```python
from build123d import *

# Parameters (mm, degrees)
F0_W     = 279.4
F0_H     = 330.2
F1_DEPTH = 5.842
F2_W     = 25.4
F2_H     = 5.842
F2_W_2   = 5.842
F2_H_2   = 25.4
F2_H_3   = 38.1
F3_DEPTH = 5.842
F5_DEPTH = 5.842
F6_W     = 5.842
F6_H     = 12.7
F7_DEPTH = 5.842
F8_R     = 3.175
F9_DEPTH = 5.842


with BuildPart() as f1:
    # F0 (on Front) → F1 (new body)
    with BuildSketch(Plane.XZ):
        with Locations((25.751306051, 40.8756073241)):
            Rectangle(F0_W, F0_H)
    extrude(amount=F1_DEPTH)

    # F2 (on face) → F3 (cut, through all)
    with BuildSketch(Plane.XZ.offset(5.842)):
        with Locations((152.751306051, -121.3033926759)):
            Rectangle(F2_W, F2_H)
        with Locations((101.951306051, -121.3033926759)):
            Rectangle(F2_W, F2_H)
        with Locations((51.151306051, -121.3033926759)):
            Rectangle(F2_W, F2_H)
        with Locations((0.351306051, -121.3033926759)):
            Rectangle(F2_W, F2_H)
        with Locations((-50.448693949, -121.3033926759)):
            Rectangle(F2_W, F2_H)
        with Locations((162.530306051, -86.1243926759)):
            Rectangle(F2_W_2, F2_H_2)
        with Locations((162.530306051, -28.9743926759)):
            Rectangle(F2_W_2, F2_H_3)
        with Locations((-111.027693949, -86.1243926759)):
            Rectangle(F2_W_2, F2_H_2)
        with Locations((-111.027693949, -35.3243926759)):
            Rectangle(F2_W_2, F2_H_2)
        with Locations((-111.027693949, 15.4756073241)):
            Rectangle(F2_W_2, F2_H_2)
        with Locations((-111.027693949, 66.2756073241)):
            Rectangle(F2_W_2, F2_H_2)
        with Locations((-111.027693949, 167.8756073241)):
            Rectangle(F2_W_2, F2_H_2)
        with Locations((-111.027693949, 117.0756073241)):
            Rectangle(F2_W_2, F2_H_2)
        with Locations((-101.248693949, -121.3033926759)):
            Rectangle(F2_W, F2_H)
    extrude(amount=-F3_DEPTH, mode=Mode.SUBTRACT)

    # F4 (on face) → F5 (cut, through all)
    with BuildSketch(Plane.XZ.offset(5.842)):
        with BuildLine():
            add(Edge.make_bspline(
                [(159.609306051, 15.4756073241), (73.376306051, 28.1756073241), (-24.4799113405, 59.233935121), (-21.873693949, 193.2756073241), (-113.948693949, 205.9756073241)],
                knots=[0, 0, 0, 0, 0.5067216409, 1, 1, 1, 1], degree=3))
            Line((159.609306051, 15.4756073241), (165.451306051, 15.4756073241))
            Line((165.451306051, 15.4756073241), (165.451306051, 205.9756073241))
            Line((165.451306051, 205.9756073241), (-113.948693949, 205.9756073241))
        make_face()
    extrude(amount=-F5_DEPTH, mode=Mode.SUBTRACT)

    # F6 (on face) → F7 (cut, through all)
    with BuildSketch(Plane.XZ.offset(5.842)):
        with Locations((162.530306051, 2.7756073241)):
            Rectangle(F6_W, F6_H)
    extrude(amount=-F7_DEPTH, mode=Mode.SUBTRACT)

    # F8 (on face) → F9 (cut, through all)
    with BuildSketch(Plane.XZ.offset(5.842)):
        with Locations((-37.748693949, 190.1641073241)):
            Circle(F8_R)
    extrude(amount=-F9_DEPTH, mode=Mode.SUBTRACT)


solid = f1.part
```
Can you work these out from the model? Positions are in its coordinate system, mm. Round coordinates to 2 decimals unless told otherwise and drop trailing zeros. Loops run counter-clockwise (first coordinate to the right, second up) from the corner with the lowest first, then second, coordinate; pieces in that order, holes last.
Item 1: Will these pins go through, and if not, where does the flat tip stop? pin 1 Ø4 at (x, z) = (53.5, 27.5) entering from +Y; pin 2 Ø1.8 at (x, y) = (161.5, -3) entering from -Z; pin 3 Ø1.8 at (x, y) = (163, -1.5) entering from +Z; pin 4 Ø1.8 at (x, y) = (-110, -2) entering from +Z.
Item 2: Suppose I cut it at A-A, the plane z = -27. Write out the boundary of the cut face in (x, y).
Item 3: Please list where these lines run through material, in increasing order: L1, parallel to X at y = -3.4, z = -3; L2, parallel to X at y = -5.1, z = -84; L3, parallel to Z at x = -8.5, y = -2.65.
Reported:
1. pin 1: stops at y = 0
1. pin 2: stops at z = -118.38
1. pin 3: stops at z = 15.48
1. pin 4: stops at z = 205.53
2. outline: (-108.11, -5.84) - (159.61, -5.84) - (159.61, 0) - (-108.11, 0) - close
3. L1: x = -113.95 to 159.61
3. L2: x = -108.11 to 159.61
3. L3: z = -118.38 to 104.32
